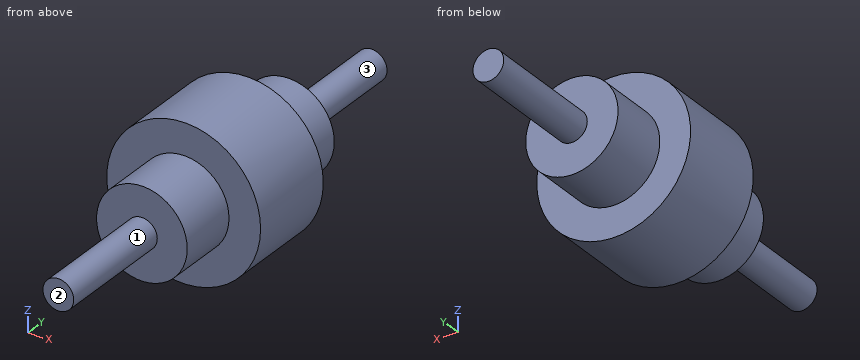
from build123d import *

# Parameters (mm, degrees)
F0_R     = 50
F1_DEPTH = 60
F2_R     = 30
F3_DEPTH = 40
F4_R     = 10
F5_DEPTH = 80
F6_R     = 29.463917
F7_DEPTH = 40
F8_R     = 10
F9_DEPTH = 80


with BuildPart() as f1:
    # F0 (on Front) → F1 (new body)
    with BuildSketch(Plane.XZ):
        Circle(F0_R)
    extrude(amount=F1_DEPTH)

    # F2 (on Front) → F3 (join)
    with BuildSketch(Plane.XZ):
        Circle(F2_R)
    extrude(amount=-F3_DEPTH)

    # F4 (on face) → F5 (join)
    with BuildSketch(Plane(origin=(0, 40, 0), x_dir=(-1, 0, 0), z_dir=(0, 1, 0))):
        Circle(F4_R)
    extrude(amount=F5_DEPTH)

    # F6 (on face) → F7 (join)
    with BuildSketch(Plane.XZ.offset(60)):
        Circle(F6_R)
    extrude(amount=F7_DEPTH)

    # F8 (on face) → F9 (join)
    with BuildSketch(Plane.XZ.offset(100)):
        Circle(F8_R)
    extrude(amount=F9_DEPTH)


solid = f1.part
The listing builds one solid part. Answer for the finished solid, in the listing's coordinates (mm). Face numbers are marked on the shaded views. A direction names the side the tool comes from. Give positions to 0.01 mm unless a question says otherwise; leave off trailing zeros. Loops run counter-clockwise (first coordinate to the right, second up) from the corner with the lowest first, then second, coordinate; pieces in that order, holes last. Notation, with made-up numbers: (12.25, 11) - (34.25, 11) arc R31 cw to (34.25, 39) - close; hole circle Ø7 at (-15.75, 37). An arc over 180 degrees is marked (long way). Use one line per item in the form item = value.
1. Given pin 1 Ø1 at (y, z) = (32.5, 26) entering from -X; pin 2 Ø2 at (x, z) = (18.5, 10) entering from +Y; pin 3 Ø6 at (x, z) = (32, -21) entering from +Y, each flat-ended and moving along its own axis, determine where each tip first touches the part or whether it passes through.
Calculated:
pin_1 = -15.8
pin_2 = 40
pin_3 = 0
2. Find the intervals of material crossed by line 1 along Y through (x, z) = (1.5, -30.5); line 2 along Y through (x, z) = (13, 10); line 3 along Z through (x, y) = (-1.5, -34.5), in increasing order. Write a range as [from, to].
Calculated:
line_1 = [-60, 0]
line_2 = [-100, 40]
line_3 = [-49.98, 49.98]
3. Section A-A on x = 0 is taken. Give the vertices of the cut face in (y, z).
Calculated:
outline = (-180, -10) - (-100, -10) - (-100, -29.46) - (-60, -29.46) - (-60, -50) - (0, -50) - (0, -30) - (40, -30) - (40, -10) - (120, -10) - (120, 10) - (40, 10) - (40, 30) - (0, 30) - (0, 50) - (-60, 50) - (-60, 29.46) - (-100, 29.46) - (-100, 10) - (-180, 10) - close
4. Section B-B on z = 0 is taken. Give the vertices of the cut face in (x, y).
Calculated:
outline = (-50, -60) - (-29.46, -60) - (-29.46, -100) - (-10, -100) - (-10, -180) - (10, -180) - (10, -100) - (29.46, -100) - (29.46, -60) - (50, -60) - (50, 0) - (30, 0) - (30, 40) - (10, 40) - (10, 120) - (-10, 120) - (-10, 40) - (-30, 40) - (-30, 0) - (-50, 0) - close
5. Which of the six approach directions +Z, -Z, +X, -X, +Y, -Y give full straight-line access (tool end or side, diameter ignored) to the marked faces 1, 2 and 3?
Calculated:
face_1 = -Y
face_2 = +Z, -Z, +X, -X, -Y
face_3 = +Y
6. Section D-D on z = 23 is taken. Give the vertices of the cut face in (x, y).
Calculated:
outline = (-44.4, -60) - (-18.42, -60) - (-18.42, -100) - (18.42, -100) - (18.42, -60) - (44.4, -60) - (44.4, 0) - (19.26, 0) - (19.26, 40) - (-19.26, 40) - (-19.26, 0) - (-44.4, 0) - close
7. Section C-C on y = 17 is taken. Give the vertices of the cut face in (x, z).
Calculated:
outline = circle Ø60 at (0, 0)
